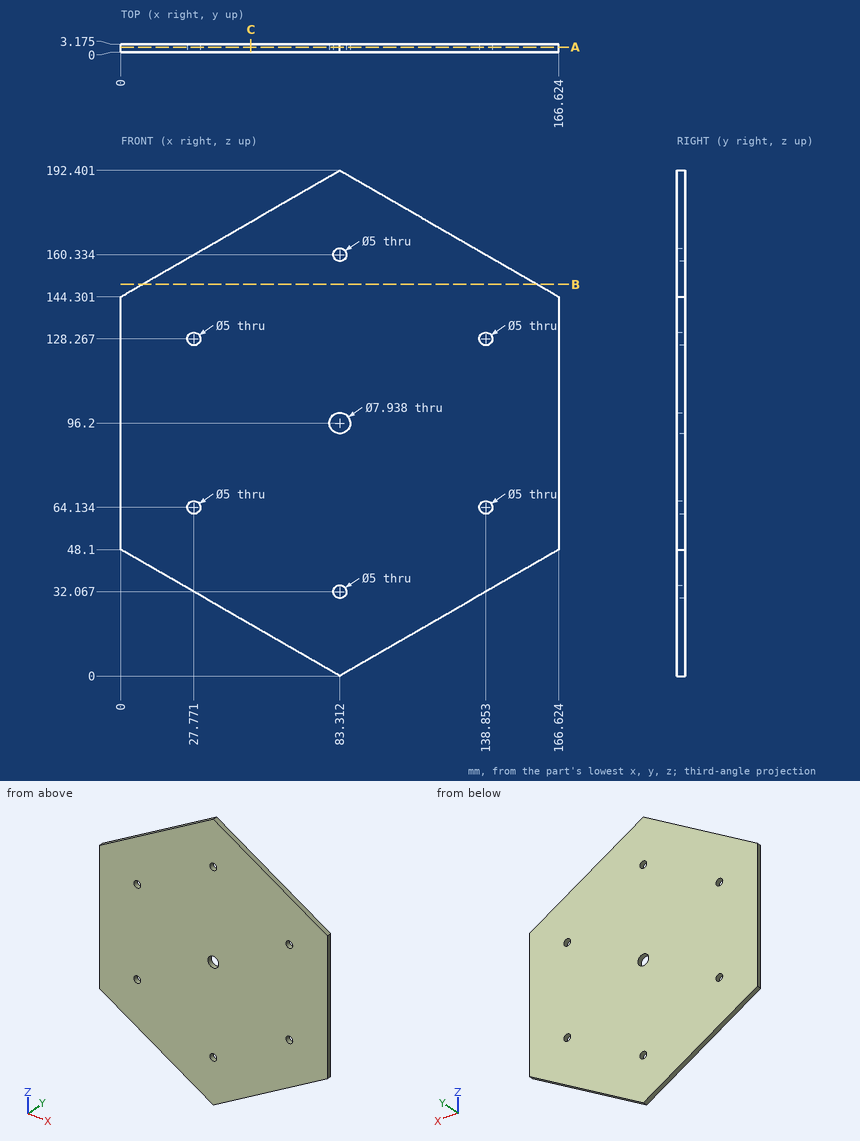
Input: dimensioned drawing with shaded views. Units: mm. Origin: part minimum x, y, z. Round coordinates to 2 decimals unless told otherwise and drop trailing zeros. Loops run counter-clockwise (first coordinate to the right, second up) from the corner with the lowest first, then second, coordinate; pieces in that order, holes last. Notation, with made-up numbers: M 29,2.5 L 87,2.5 A11 ccw 87,23.5 Z; hole C 12,74.25 d1. An arc over 180 degrees is marked long. Return JSON: item names as keys, results as strings. Group by question number.
1. Material intervals for line 1 along X through (y, z) = (2.4, 96) (1 decimal); line 2 along Z through (x, y) = (137, 2.4) (1 decimal); line 3 along X through (y, z) = (2.8, 65) (1 decimal), sorted ascending. Write a range as from..to.
2. Section query A-A on y = 2. Output: boundary loops of the cut face in (x, z) (1 decimal).
3. Section query C-C on x = 49.5. Output: boundary loops of the cut face in (y, z) (1 decimal), and give its area (3 significant figures).
4. Pin query (flat end, axial travel): pin 1 (4 mm diameter, centred on x = 138.85, z = 128.27, fed in from -Y). Return the tip coordinate at first contact, or that it passes through.
5. Section query B-B on z = 149. Output: boundary loops of the cut face in (x, y) (1 decimal).
Checks:
{
 "1": {"line 1": "x = 0..79.3, 87.3..166.6", "line 2": "z = 31..62.5, 65.8..126.6, 129.9..161.4", "line 3": "x = 0..25.4, 30.1..136.5, 141.2..166.6"},
 "2": {"outline": "M 0,48.1 L 83.3,0 L 166.6,48.1 L 166.6,144.3 L 83.3,192.4 L 0,144.3 Z; hole C 27.8,64.1 d5; hole C 27.8,128.3 d5; hole C 83.3,96.2 d7.9; hole C 83.3,32.1 d5; hole C 83.3,160.3 d5; hole C 138.9,64.1 d5; hole C 138.9,128.3 d5"},
 "3": {"outline": "M 0,19.5 L 3.2,19.5 L 3.2,172.9 L 0,172.9 Z", "area": "487 mm²"},
 "4": {"pin 1": "passes through"},
 "5": {"outline": "M 8.1,0 L 158.5,0 L 158.5,3.2 L 8.1,3.2 Z"}
}
